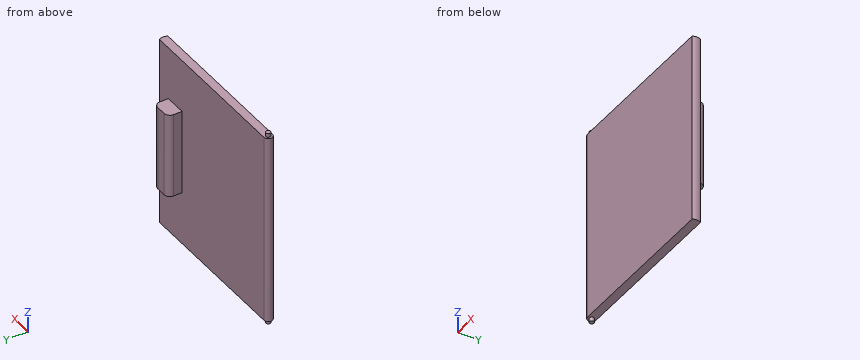
from build123d import *

# Parameters (mm, degrees)
BOSS_EXTRUDE1_DEPTH = 67.5
SKETCH2_R           = 0.8
BOSS_EXTRUDE2_DEPTH = 1.375
BOSS_EXTRUDE3_START = 1.375
SKETCH3_R           = 0.8
BOSS_EXTRUDE3_DEPTH = 1.375
BOSS_EXTRUDE4_DEPTH = 67.5
SKETCH5_W           = 7.5
SKETCH5_H           = 30
BOSS_EXTRUDE5_DEPTH = 5
FILLET1_R           = 2


with BuildPart() as part:
    # Sketch1 → Boss-Extrude1 (new body)
    with BuildSketch(Plane.XY):
        with BuildLine():
            Line((0, -1.5), (57.5, -1.5))
            Line((57.5, -1.5), (57.5, 1.5))
            Line((57.5, 1.5), (0, 1.5))
            ThreePointArc((0, 1.5), (-1.5, 0), (0, -1.5))
        make_face()
    extrude(amount=BOSS_EXTRUDE1_DEPTH)

    # Sketch2 → Boss-Extrude2 (add)
    with BuildSketch(Plane.XY.offset(67.5)):
        Circle(SKETCH2_R)
    extrude(amount=BOSS_EXTRUDE2_DEPTH)

    # Sketch3 → Boss-Extrude3 (add)
    with BuildSketch(Plane(origin=(0, 0, 0), x_dir=(-1, 0, 0), z_dir=(0, 0, -1)).offset(BOSS_EXTRUDE3_START)):
        with Locations(Location((0, 0, 0), (0, 0, 180))):
            Circle(SKETCH3_R)
    extrude(amount=-BOSS_EXTRUDE3_DEPTH)

    # Sketch4 → Boss-Extrude4 (add)
    with BuildSketch(Plane.XY.offset(67.5)):
        with BuildLine():
            Line((57.5, 1.5), (57.5, -1.5))
            ThreePointArc((57.5, -1.5), (57.854101966, 0), (57.5, 1.5))
        make_face()
    extrude(amount=-BOSS_EXTRUDE4_DEPTH)

    # Sketch5 → Boss-Extrude5 (add)
    with BuildSketch(Plane(origin=(0, 1.5, 0), x_dir=(1, 0, 0), z_dir=(0, 1, 0))):
        with Locations((48.75, -33.75)):
            Rectangle(SKETCH5_W, SKETCH5_H)
    extrude(amount=BOSS_EXTRUDE5_DEPTH)

    # Fillet1
    fillet1_edges = [part.edges().sort_by_distance(p)[0] for p in [
        (45, 6.5, 33.75),
        (52.5, 6.5, 33.75),
    ]]
    fillet(fillet1_edges, radius=FILLET1_R)


solid = part.part
Model file for the job. Use its own axes, mm. Give positions to 0.01 mm unless a question says otherwise; leave off trailing zeros. Loops run counter-clockwise (first coordinate to the right, second up) from the corner with the lowest first, then second, coordinate; pieces in that order, holes last.
1) Wall check: line 1 (Y direction, x = 29, z = 39.5); line 2 (X direction, y = 2.75, z = 35); line 3 (Z direction, x = 20, y = 1). Give the ranges that are in metal, low to high.
2) Saw through at D-D (z = 17.5). Write the cut outline in (x, y), plus the area to 3 significant figures.
3) Saw through at A-A (y = 0). Write the cut outline in (x, z) (3 decimals).
4) Flat gauge pins, fed straight in: pin 1 Ø1.5 at (y, z) = (2.5, 38) entering from -X; pin 2 Ø3.5 at (y, z) = (2.5, 29) entering from +X; pin 3 Ø2.5 at (x, y) = (24, 0.5) entering from -Z. Where does each tip first touch, or does it go through?
5) Saw through at B-B (z = 30). Write the cut outline in (x, y), plus the area to 3 significant figures.
6) Saw through at C-C (x = 40.5). Write the cut outline in (y, z).
Answer block:
1. line 1: y = -1.5 to 1.5
1. line 2: x = 45 to 52.5
1. line 3: z = 0 to 67.5
2. outline: (0, -1.5) - (57.5, -1.5) arc R3.35 ccw to (57.5, 1.5) - (0, 1.5) arc R1.5 ccw to start
2. area: 177 mm2
3. outline: (-1.5, 0) - (-0.8, 0) - (-0.8, -1.375) - (0.8, -1.375) - (0.8, 0) - (57.854, 0) - (57.854, 67.5) - (0.8, 67.5) - (0.8, 68.875) - (-0.8, 68.875) - (-0.8, 67.5) - (-1.5, 67.5) - close
4. pin 1: stops at x = 45
4. pin 2: stops at x = 57.77
4. pin 3: stops at z = 0
5. outline: (0, -1.5) - (57.5, -1.5) arc R3.35 ccw to (57.5, 1.5) - (52.5, 1.5) - (52.5, 4.5) arc R2 ccw to (50.5, 6.5) - (47, 6.5) arc R2 ccw to (45, 4.5) - (45, 1.5) - (0, 1.5) arc R1.5 ccw to start
5. area: 213 mm2
6. outline: (-1.5, 0) - (1.5, 0) - (1.5, 67.5) - (-1.5, 67.5) - close
